```python
from build123d import *

# Parameters (mm, degrees)
SKETCH_1_R            = 8
EXTRUDE_1_DEPTH       = 10
SKETCH_9_W            = 7.120641766
SKETCH_9_H            = 4.534999238
EXTRUDE_6_DEPTH       = 1
SKETCH_11_W           = 1.257653538
SKETCH_11_H           = 9
EXTRUDE_7_DEPTH       = 4.5
EXTRUDE_8_DEPTH       = 6
FILLET_8_R            = 1
FILLET_9_R            = 1
CUT_EXTRUDE_1_DEPTH   = 10
SKETCH_14_W           = 1
SKETCH_14_H           = 3
EXTRUDE_9_DEPTH       = 3.122043073
SKETCH_15_W           = 1
SKETCH_15_H           = 3
EXTRUDE_10_DEPTH      = 4
EXTRUDE_11_DEPTH      = 0.2
EXTRUDE_11_DEPTH_BACK = 1.043632387
SKETCH_16_W           = 9.952294967
SKETCH_16_H           = 3.01746433
FILLET_11_R           = 1
FILLET_12_R           = 1
FILLET_13_R           = 1
FILLET_14_R           = 1
CUT_EXTRUDE_2_DEPTH   = 10
SKETCH_18_W           = 2.361428176
SKETCH_18_H           = 7.68123899
CUT_EXTRUDE_3_DEPTH   = 10
SKETCH_19_W           = 2.115065294
SKETCH_19_H           = 7.68123899
CUT_EXTRUDE_4_DEPTH   = 2
SKETCH_20_W           = 2.115065294
SKETCH_20_H           = 7.649055087
CUT_EXTRUDE_5_DEPTH   = 2
FILLET_15_R           = 1
FILLET_16_R           = 1
FILLET_17_R           = 1
FILLET_18_R           = 1


with BuildPart() as part:
    # Sketch 1 → Extrude 1 (new body)
    with BuildSketch(Plane(origin=(0.382706605, 0, 0), x_dir=(1, 0, 0), z_dir=(0, 0, 1))):
        with Locations((-75.594417438, 2.55)):
            Circle(SKETCH_1_R)
    extrude(amount=EXTRUDE_1_DEPTH)

    # Sketch 9 → Extrude 6 (add)
    with BuildSketch(Plane(origin=(6.127831546, 0, 9), x_dir=(1, 0, 0), z_dir=(0, 0, 1))):
        with Locations((-75.644850643, 2.267499619)):
            Rectangle(SKETCH_9_W, SKETCH_9_H)
    extrude(amount=EXTRUDE_6_DEPTH)



with BuildPart() as body_2:
    # Sketch 11 → Extrude 7 (new body)
    with BuildSketch(Plane(origin=(9.574526933, 4.534999238, 0.48426017), x_dir=(1, 0, 0), z_dir=(0, 1, 0))):
        with Locations((-76.184774061, -4.5)):
            Rectangle(SKETCH_11_W, SKETCH_11_H)
    extrude(amount=-EXTRUDE_7_DEPTH)


with BuildPart() as part_1:
    add(part.part)

    add(body_2.part)  # Extrude 8 merges body 2
    # Sketch 12 → Extrude 8 (add)
    with BuildSketch(Plane.ZY.offset(67.239073897)):
        Polygon((0.48426017, 4.534999238), (0.48426017, 0), (1.483647509, 0.034999238), (1.483647509, 4.534999238), align=None)
    extrude(amount=EXTRUDE_8_DEPTH)

    # Fillet 8
    fillet_8_edges = [part_1.edges().sort_by_distance(p)[0] for p in [
        (-65.981420359, 2.284999238, 0.48426017),
    ]]
    fillet(fillet_8_edges, radius=FILLET_8_R)

    # Fillet 9
    fillet_9_edges = [part_1.edges().sort_by_distance(p)[0] for p in [
        (-65.956698214, 2.267499619, 10),
    ]]
    fillet(fillet_9_edges, radius=FILLET_9_R - 0.0001)  # a hair under: the kernel refuses the full size

    # Sketch 13 → Cut-Extrude 1 (cut)
    with BuildSketch(Plane(origin=(0, 0, 0), x_dir=(-1, 0, 0), z_dir=(0, 0, -1))):
        with BuildLine():
            Line((69.041558468, 7.642074214), (69.041558468, -2.542074214))
            ThreePointArc((69.041558468, -2.542074214), (63.949484255, 2.55), (69.041558468, 7.642074214))
        make_face()
    extrude(amount=-CUT_EXTRUDE_1_DEPTH, mode=Mode.SUBTRACT)

    # Sketch 14 → Extrude 9 (add)
    with BuildSketch(Plane(origin=(-69.041558468, 0, 0), x_dir=(0, 0, -1), z_dir=(1, 0, 0))):
        with Locations((-9.5, 2.417510407)):
            Rectangle(SKETCH_14_W, SKETCH_14_H)
    extrude(amount=EXTRUDE_9_DEPTH)

    # Sketch 15 → Extrude 10 (add)
    with BuildSketch(Plane(origin=(-69.041558468, 0, 0), x_dir=(0, 0, -1), z_dir=(1, 0, 0))):
        with Locations((-0.5, 2.417510407)):
            Rectangle(SKETCH_15_W, SKETCH_15_H)
    extrude(amount=EXTRUDE_10_DEPTH)

    # Sketch 16 → Extrude 11 (add, two sides: drawn at the far end of the back side and taken through both)
    with BuildSketch(Plane(origin=(-65.041558468, 0, 0), x_dir=(0, 0, -1), z_dir=(1, 0, 0)).offset(-EXTRUDE_11_DEPTH_BACK)):
        with Locations((-4.976147484, 2.408778242)):
            Rectangle(SKETCH_16_W, SKETCH_16_H)
    extrude(amount=EXTRUDE_11_DEPTH + EXTRUDE_11_DEPTH_BACK)

    # Fillet 11
    fillet_11_edges = [part_1.edges().sort_by_distance(p)[0] for p in [
        (-64.841558468, 2.408778242, 0),
    ]]
    fillet(fillet_11_edges, radius=FILLET_11_R)

    # Fillet 12
    fillet_12_edges = [part_1.edges().sort_by_distance(p)[0] for p in [
        (-64.841558468, 2.408778242, 9.952294967),
    ]]
    fillet(fillet_12_edges, radius=FILLET_12_R)

    # Fillet 13
    fillet_13_edges = [part_1.edges().sort_by_distance(p)[0] for p in [
        (-69.041558468, 7.642074214, 5),
    ]]
    fillet(fillet_13_edges, radius=FILLET_13_R)

    # Fillet 14
    fillet_14_edges = [part_1.edges().sort_by_distance(p)[0] for p in [
        (-69.041558468, -2.542074214, 5),
    ]]
    fillet(fillet_14_edges, radius=FILLET_14_R)

    # Sketch 17 → Cut-Extrude 2 (cut)
    with BuildSketch(Plane(origin=(0, 0, 0), x_dir=(-1, 0, 0), z_dir=(0, 0, -1))):
        with BuildLine():
            Line((81.390220844, 7.631930149), (81.390220844, -2.531930149))
            ThreePointArc((81.390220844, -2.531930149), (84.200552216, 2.55), (81.390220844, 7.631930149))
        make_face()
    extrude(amount=-CUT_EXTRUDE_2_DEPTH, mode=Mode.SUBTRACT)

    # Sketch 18 → Cut-Extrude 3 (cut)
    with BuildSketch(Plane(origin=(0, 0, 0), x_dir=(-1, 0, 0), z_dir=(0, 0, -1))):
        with Locations((78.094441462, 2.579171883)):
            Rectangle(SKETCH_18_W, SKETCH_18_H)
    extrude(amount=-CUT_EXTRUDE_3_DEPTH, mode=Mode.SUBTRACT)

    # Sketch 19 → Cut-Extrude 4 (cut)
    with BuildSketch(Plane(origin=(0, 0, 0), x_dir=(-1, 0, 0), z_dir=(0, 0, -1))):
        with Locations((80.332688197, 2.579171883)):
            Rectangle(SKETCH_19_W, SKETCH_19_H)
    extrude(amount=-CUT_EXTRUDE_4_DEPTH, mode=Mode.SUBTRACT)

    # Sketch 20 → Cut-Extrude 5 (cut)
    with BuildSketch(Plane.XY.offset(10)):
        with Locations((-80.332688197, 2.595263834)):
            Rectangle(SKETCH_20_W, SKETCH_20_H)
    extrude(amount=-CUT_EXTRUDE_5_DEPTH, mode=Mode.SUBTRACT)

    # Fillet 15
    fillet_15_edges = [part_1.edges().sort_by_distance(p)[0] for p in [
        (-81.390220844, 7.025860764, 0),
    ]]
    fillet(fillet_15_edges, radius=FILLET_15_R)

    # Fillet 16
    fillet_16_edges = [part_1.edges().sort_by_distance(p)[0] for p in [
        (-81.390220844, 7.025860764, 10),
    ]]
    fillet(fillet_16_edges, radius=FILLET_16_R)

    # Fillet 17
    fillet_17_edges = [part_1.edges().sort_by_distance(p)[0] for p in [
        (-81.390220844, -1.89668888, 0),
    ]]
    fillet(fillet_17_edges, radius=FILLET_17_R)

    # Fillet 18
    fillet_18_edges = [part_1.edges().sort_by_distance(p)[0] for p in [
        (-81.390220844, -1.880596929, 10),
    ]]
    fillet(fillet_18_edges, radius=FILLET_18_R)


solid = part_1.part
```
Model file for the job. Use its own axes, mm. A direction names the side the tool comes from. Coordinates: 2 decimals unless noted, no trailing zeros. Order: outer loops, then holes, each group sorted by start corner. A loop starts at its lowest first (then second) coordinate and runs counter-clockwise, first axis right, second up. Notation, with made-up numbers: (83.5, -5.5) - (141.5, -5.5) arc R23 cw to (141.5, 13.5) - close; hole circle Ø5 at (81, 13.25). An arc over 180 degrees is marked (long way). Return JSON: item names as keys, results as strings. Group by question number.
1) Saw through at C-C, the plane x = -77.25. Write the cut outline in (y, z), plus the area to 3 significant figures.
2) Saw through at A-A, the plane y = 1.25. Write the cut outline in (x, z), plus the area to 3 significant figures.
3) Probe line 1 (X direction, y = 3.25, z = 6.25); line 2 (Z direction, x = -67.75, y = 1.5); line 3 (X direction, y = 1, z = 1.5). List the from-to ranges inside material, lowest first. Write a range as from..to.
4) Saw through at B-B, the plane z = 7.25. Write the cut outline in (x, y), plus the area to 3 significant figures.
5) Tool access for faces 1 (the flat face through (-79, -1.261, 4)), 2 (the flat face through (-65, 0.9, 5)), 3 (the flat face through (-79.275, 3, 5)), 4 (the flat face through (-68, 2, 9)): list every direction of +Z, -Z, +X, -X, +Y, -Y with a clear straight run to the whole face (end or side of a thin tool).
6) Flat gauge pins, fed straight in: P1, Ø0.5, axis at x = -67.5, z = 0.5, coming from the -Y side; P2, Ø8, axis at x = -68, y = 8.5, coming from the +Z side; P3, Ø2, axis at x = -66.5, z = 2.5, coming from the +Y side; P4, Ø1, axis at x = -79.5, z = 8, coming from the -Y side. Where does each tip first touch, or does it go through?
7) Mould opens along X. For faces 5 (the cylindrical face through (-65.14, 2.43, 0.29)), 6 (the flat face through (-67.5, 0.918, 9.5)), 7 (the flat face through (-80, 3, 8)) say: released by +X, released by -X, zero draft, split by the parting line, or undercut.
Values found:
{
 "1": {"outline": "(-5.19, 0) - (-1.26, 0) - (-1.26, 10) - (-5.19, 10) - close; (6.42, 0) - (10.29, 0) - (10.29, 10) - (6.42, 10) - close", "area": "77.9 mm²"},
 "2": {"outline": "(-81.39, 2) - (-79.28, 2) - (-79.28, 8) - (-81.39, 8) - close; (-76.91, 0) - (-65.84, 0) arc R1 ccw to (-64.84, 1) - (-64.84, 8.95) arc R1 ccw to (-65.84, 9.95) - (-65.92, 9.95) - (-65.92, 10) - (-76.91, 10) - close; hole (-69.04, 1) - (-66.09, 1) - (-66.09, 9) - (-69.04, 9) - close", "area": "109 mm²"},
 "3": {"line 1": "x = -81.39..-79.28, -76.91..-69.04, -66.09..-64.84", "line 2": "z = 0..1, 9..10", "line 3": "x = -76.91..-69.04, -66.09..-64.84"},
 "4": {"outline": "(-81.39, -2.53) arc R8 ccw to (-69.3, -2.84) arc R1 ccw to (-69.04, -2.17) - (-69.04, 7.27) arc R1 ccw to (-69.3, 7.94) arc R8 ccw to (-81.39, 7.63) - close; (-66.09, 0.9) - (-64.84, 0.9) - (-64.84, 3.92) - (-66.09, 3.92) - close; hole (-79.28, -1.26) - (-76.91, -1.26) - (-76.91, 6.42) - (-79.28, 6.42) - close", "area": "161 mm²"},
 "5": {"face 1": "-Z", "face 2": "+Z, -Z, +X, -Y", "face 3": "+Z, -Z", "face 4": "+Y, -Y"},
 "6": {"P1": "stops at y = 0.92", "P2": "stops at z = 10", "P3": "stops at y = 3.92", "P4": "stops at y = -4.5"},
 "7": {"face 5": "released by +X", "face 6": "undercut", "face 7": "zero draft"}
}
